Geometry: final body of the model. Coordinates: model frame, mm. Face numbers are marked on the shaded views. A direction names the side the tool comes from. Coordinates: 2 decimals unless noted, no trailing zeros. Loops run counter-clockwise (first coordinate to the right, second up) from the corner with the lowest first, then second, coordinate; pieces in that order, holes last. Notation, with made-up numbers: (34.25, -7.75) - (47.25, -7.75) arc R15 ccw to (47.25, 9.25) - close; hole circle Ø7 at (11.5, 86). An arc over 180 degrees is marked (long way). Return JSON: item names as keys, results as strings.
from build123d import *

# Parameters (mm, degrees)
SKETCH1_R           = 1.55
BOSS_EXTRUDE1_DEPTH = 9.525
CUT_EXTRUDE1_DEPTH  = 5.9
FILLET1_R           = 0.508


with BuildPart() as part:
    # Sketch1 → Boss-Extrude1 (new body)
    # profile 1 of 5: a face of its own
    with BuildSketch(Plane(origin=(0, 0, 0), x_dir=(1, 0, 0), z_dir=(0, 1, 0))):
        Polygon((0, -6), (0, 0), (-7.245, 0), (-7.245, -8.54), (0.375, -8.54), (0.375, -6), align=None)
        with Locations(Location((-3.6225, -4.27, 0), (0, 0, 90))):
            Circle(SKETCH1_R, mode=Mode.SUBTRACT)
    # profile 2 of 5: a face of its own
    with BuildSketch(Plane(origin=(0, 0, 0), x_dir=(1, 0, 0), z_dir=(0, 1, 0))):
        Polygon((12.9, -6), (12.9, 0), (0, 0), (0, -6), (0.375, -6), (0.375, -8.54), (12.525, -8.54), (12.525, -6), align=None)
    # profile 3 of 5: a face of its own
    with BuildSketch(Plane(origin=(0, 0, 0), x_dir=(1, 0, 0), z_dir=(0, 1, 0))):
        Polygon((20.145, 0), (12.9, 0), (12.9, -6), (12.525, -6), (12.525, -8.54), (20.145, -8.54), align=None)
        with Locations(Location((16.5225, -4.27, 0), (0, 0, 90))):
            Circle(SKETCH1_R, mode=Mode.SUBTRACT)
    # profile 4 of 5: a face of its own
    with BuildSketch(Plane(origin=(0, 0, 0), x_dir=(1, 0, 0), z_dir=(0, 1, 0))):
        Polygon((0, -6), (0, 0), (-7.245, 0), (-7.245, -8.54), (0.375, -8.54), (0.375, -6), align=None)
        with Locations(Location((-3.6225, -4.27, 0), (0, 0, 90))):
            Circle(SKETCH1_R, mode=Mode.SUBTRACT)
    # profile 5 of 5: a face of its own
    with BuildSketch(Plane(origin=(0, 0, 0), x_dir=(1, 0, 0), z_dir=(0, 1, 0))):
        Polygon((20.145, 0), (12.9, 0), (12.9, -6), (12.525, -6), (12.525, -8.54), (20.145, -8.54), align=None)
        with Locations(Location((16.5225, -4.27, 0), (0, 0, 90))):
            Circle(SKETCH1_R, mode=Mode.SUBTRACT)
    extrude(amount=BOSS_EXTRUDE1_DEPTH)

    # Sketch1<4> → Cut-Extrude1 (cut)
    with BuildSketch(Plane(origin=(0, 0, 0), x_dir=(1, 0, 0), z_dir=(0, 1, 0))):
        Polygon((12.9, -6), (12.9, 0), (0, 0), (0, -6), (0.375, -6), (0.375, -8.54), (12.525, -8.54), (12.525, -6), align=None)
    extrude(amount=CUT_EXTRUDE1_DEPTH, mode=Mode.SUBTRACT)

    # Fillet1
    fillet1_edges = [part.edges().sort_by_distance(p)[0] for p in [
        (-7.245, 9.525, 4.27),
        (20.145, 9.525, 4.27),
    ]]
    fillet(fillet1_edges, radius=FILLET1_R)


solid = part.part
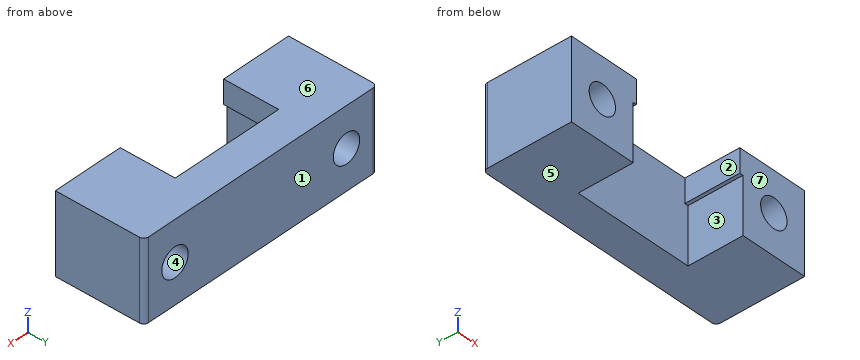
Item 1: Mould query, pull axis Z, two halves, no side actions, for the marked faces 4, 5, 6 and 7. Classes: +Z half, -Z half, draft (parallel to the pull), parting line (faces both ways), or undercut.
Worked out:
{"face 4": "undercut", "face 5": "-Z half", "face 6": "+Z half", "face 7": "draft"}
Item 2: Section query A-A, the plane y = 1.5. Count the separate pieces of the cut face and the enclosed holes in it, and give its area (3 significant figures).
Worked out:
{"separate pieces": "2", "enclosed holes": "2", "area": "111 mm^2"}
Item 3: Reachability of the marked faces 1, 2 and 3 from +Z, -Z, +X, -X, +Y, -Y: full face, straight path, thin tool, end or side. Return the list, or none.
Worked out:
{"face 1": "+Z, -Z, +X, -X, +Y", "face 2": "+Z, -Z, -Y", "face 3": "-Z, -Y"}
Item 4: First-contact query: pin 1 Ø5 at (x, z) = (16.52, 4.27) entering from -Y; pin 2 Ø3 at (x, z) = (5, 2.5) entering from -Y. Flat tips, straight axial feed; report the tip coordinate or a pass-through.
Worked out:
{"pin 1": "y = 0", "pin 2": "y = 5.9"}
Item 5: Section query B-B, the plane z = 4.27. Return loops of the section in (x, y) (1 decimal), and give its area (3 significant figures).
Worked out:
{"outline": "(-7.2, 0) - (-5.2, 0) - (-5.2, 9.5) - (-6.7, 9.5) arc R0.5 ccw to (-7.2, 9) - close; (-2.1, 0) - (0, 0) - (0, 5.9) - (12.9, 5.9) - (12.9, 0) - (15, 0) - (15, 9.5) - (-2.1, 9.5) - close; (18.1, 0) - (20.1, 0) - (20.1, 9) arc R0.5 ccw to (19.6, 9.5) - (18.1, 9.5) - close", "area": "126 mm^2"}
Item 6: Section query C-C, the plane x = -4. Return loops of the section in (y, z) (3 decimals).
Worked out:
{"outline": "(0, 0) - (9.525, 0) - (9.525, 2.767) - (0, 2.767) - close; (0, 5.773) - (9.525, 5.773) - (9.525, 8.54) - (0, 8.54) - close"}
Item 7: Ray query, probe 1 along X at (y, z) = (4.25, 4.27) (1 decimal); probe 2 along X at (y, z) = (6.5, 4.27) (1 decimal); probe 3 along X at (y, z) = (2, 1.75) (3 decimals). Return the intervals inside material, ascending. Write a range as from..to.
Worked out:
{"probe 1": "-7.2..-5.2, -2.1..0, 12.9..15, 18.1..20.1", "probe 2": "-7.2..-5.2, -2.1..15, 18.1..20.1", "probe 3": "-7.245..0, 12.9..20.145"}
